```python
from build123d import *

# Parameters (mm, degrees)
SKETCH008_W     = 110
SKETCH008_H     = 66
PAD006_DEPTH    = 2
SKETCH010_W     = 110
SKETCH010_H     = 66
PAD008_DEPTH    = 40
SKETCH011_W     = 106
SKETCH011_H     = 62
POCKET003_DEPTH = 40
SKETCH012_W     = 8
SKETCH012_H     = 8
PAD009_DEPTH    = 38
FILLET_R        = 2
FILLET001_R     = 2
FILLET002_R     = 2
FILLET003_R     = 2
FILLET004_R     = 2
SKETCH009_R     = 3
PAD010_DEPTH    = 10
SKETCH013_W     = 16
SKETCH013_H     = 10
POCKET004_DEPTH = 2
SKETCH014_R     = 1
POCKET005_DEPTH = 8
FILLET005_R     = 1
FILLET006_R     = 1
FILLET007_R     = 2
SKETCH015_R     = 1
POCKET006_DEPTH = 5
FILLET008_R     = 1
SKETCH016_W     = 12
SKETCH016_H     = 2
PAD011_DEPTH    = 38


with BuildPart() as part:
    # Sketch008 → Pad006 (new body)
    with BuildSketch(Plane.XY):
        with Locations((9, 0)):
            Rectangle(SKETCH008_W, SKETCH008_H)
    extrude(amount=PAD006_DEPTH)

    # Sketch010 (on Face6 of Pad006) → Pad008 (join)
    with BuildSketch(Plane.XY.offset(2)):
        with Locations((9, 0)):
            Rectangle(SKETCH010_W, SKETCH010_H)
    extrude(amount=PAD008_DEPTH)

    # Sketch011 (on Face9 of Pad008) → Pocket003 (cut)
    with BuildSketch(Plane.XY.offset(42)):
        with Locations((9, 0)):
            Rectangle(SKETCH011_W, SKETCH011_H)
    extrude(amount=-POCKET003_DEPTH, mode=Mode.SUBTRACT)

    # Sketch012 (on Face15 of Pocket003) → Pad009 (join)
    with BuildSketch(Plane.XY.offset(2)):
        with Locations((-40, 27)):
            Rectangle(SKETCH012_W, SKETCH012_H)
        with Locations((58, 27)):
            Rectangle(SKETCH012_W, SKETCH012_H)
        with Locations((-40, -27)):
            Rectangle(SKETCH012_W, SKETCH012_H)
        with Locations((58, -27)):
            Rectangle(SKETCH012_W, SKETCH012_H)
    extrude(amount=PAD009_DEPTH)

    # Fillet
    fillet_edges = [part.edges().sort_by_distance(p)[0] for p in [
        (62, -31, 41),
    ]]
    fillet(fillet_edges, radius=FILLET_R)

    # Fillet001
    fillet001_edges = [part.edges().sort_by_distance(p)[0] for p in [
        (-44, 31, 41),
    ]]
    fillet(fillet001_edges, radius=FILLET001_R)

    # Fillet002
    fillet002_edges = [part.edges().sort_by_distance(p)[0] for p in [
        (62, 31, 41),
    ]]
    fillet(fillet002_edges, radius=FILLET002_R)

    # Fillet003
    fillet003_edges = [part.edges().sort_by_distance(p)[0] for p in [
        (-44, -31, 41),
    ]]
    fillet(fillet003_edges, radius=FILLET003_R)

    # Fillet004
    fillet004_edges = [part.edges().sort_by_distance(p)[0] for p in [
        (64, 33, 22),
        (64, -33, 22),
        (-46, -33, 22),
        (-46, 33, 22),
    ]]
    fillet(fillet004_edges, radius=FILLET004_R)

    # Sketch009 → Pad010 (join)
    with BuildSketch(Plane.XY.offset(2)):
        with Locations((-38, 18.5)):
            Circle(SKETCH009_R)
        with Locations((45, 18.5)):
            Circle(SKETCH009_R)
        with Locations((-38, -18.5)):
            Circle(SKETCH009_R)
        with Locations((45, -18.5)):
            Circle(SKETCH009_R)
    extrude(amount=PAD010_DEPTH)

    # Sketch013 (on Face5 of Pad010) → Pocket004 (cut)
    with BuildSketch(Plane(origin=(-46, 0, 0), x_dir=(0, -1, 0), z_dir=(-1, 0, 0))):
        with Locations((0, 12)):
            Rectangle(SKETCH013_W, SKETCH013_H)
    extrude(amount=-POCKET004_DEPTH, mode=Mode.SUBTRACT)

    # Sketch014 (on Face35 of Pocket004) → Pocket005 (cut)
    with BuildSketch(Plane.XY.offset(40)):
        with Locations((-40, 27)):
            Circle(SKETCH014_R)
        with Locations((58, 27)):
            Circle(SKETCH014_R)
        with Locations((-40, -27)):
            Circle(SKETCH014_R)
        with Locations((58, -27)):
            Circle(SKETCH014_R)
    extrude(amount=-POCKET005_DEPTH, mode=Mode.SUBTRACT)

    # Fillet005
    fillet005_edges = [part.edges().sort_by_distance(p)[0] for p in [
        (9, 33, 42),
        (63.414214, 32.414214, 42),
        (64, 0, 42),
        (-45.414214, 32.414214, 42),
        (-46, 0, 42),
        (-45.414214, -32.414214, 42),
        (9, -33, 42),
        (63.414214, -32.414214, 42),
    ]]
    fillet(fillet005_edges, radius=FILLET005_R)

    # Fillet006
    fillet006_edges = [part.edges().sort_by_distance(p)[0] for p in [
        (-45, -8, 17),
        (-45, 8, 7),
        (-45, 8, 17),
        (-45, -8, 7),
    ]]
    fillet(fillet006_edges, radius=FILLET006_R)

    # Fillet007
    fillet007_edges = [part.edges().sort_by_distance(p)[0] for p in [
        (54, 23, 21),
        (54, -23, 21),
        (-36, 23, 21),
        (-36, -23, 21),
    ]]
    fillet(fillet007_edges, radius=FILLET007_R)

    # Sketch015 (on Face55 of Fillet007) → Pocket006 (cut)
    with BuildSketch(Plane.XY.offset(12)):
        with Locations((-38, 18.5)):
            Circle(SKETCH015_R)
        with Locations((45, 18.5)):
            Circle(SKETCH015_R)
        with Locations((-38, -18.5)):
            Circle(SKETCH015_R)
        with Locations((45, -18.5)):
            Circle(SKETCH015_R)
    extrude(amount=-POCKET006_DEPTH, mode=Mode.SUBTRACT)

    # Fillet008
    fillet008_edges = [part.edges().sort_by_distance(p)[0] for p in [
        (-46, 8, 12),
        (-46, 7.707107, 7.292893),
        (-46, 7.707107, 16.707107),
        (-46, 0, 17),
        (-46, -7.707107, 16.707107),
        (-46, -8, 12),
        (-46, -7.707107, 7.292893),
        (-46, 0, 7),
    ]]
    fillet(fillet008_edges, radius=FILLET008_R)

    # Sketch016 (on Face21 of Fillet008) → Pad011 (join)
    with BuildSketch(Plane.XY.offset(2)):
        with Locations((9, 30)):
            Rectangle(SKETCH016_W, SKETCH016_H)
        with Locations((9, -30)):
            Rectangle(SKETCH016_W, SKETCH016_H)
    extrude(amount=PAD011_DEPTH)


solid = part.part
```
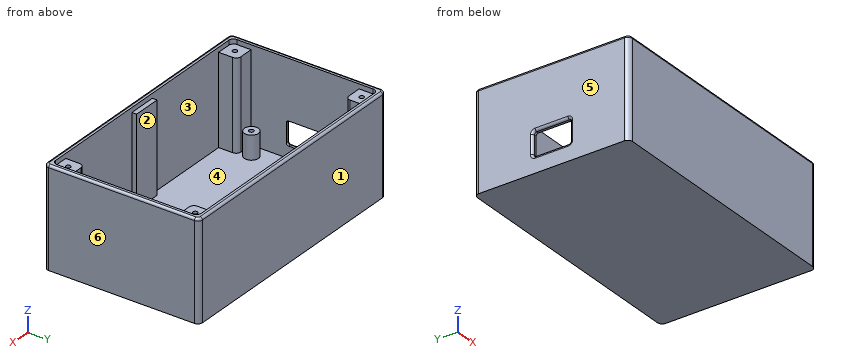
Work out the finished part from the listing and answer in its coordinate system (mm). Face numbers are marked on the shaded views. A direction names the side the tool comes from. Round coordinates to 2 decimals unless told otherwise and drop trailing zeros. Loops run counter-clockwise (first coordinate to the right, second up) from the corner with the lowest first, then second, coordinate; pieces in that order, holes last. Notation, with made-up numbers: (-23, 13) -> (21, 13) arc R31 ccw to (21, 46) -> close; hole circle Ø2 at (66.25, 49.25). An arc over 180 degrees is marked (long way). Write each question's results on one line, items separated by ' | '. Start each with the question number.
1. A tool of negligible diameter and unlimited length cuts with its end or side. For the marked faces 1 and 2, from which of +Z, -Z, +X, -X, +Y, -Y can it reach the whole face along a straight path? Write none if from no direction.
2. Section B-B (x = 32.5) is taken. Determine the outline of the cut face in (y, z), plus the area to 3 significant figures.
3. Find the intervals of material crossed by probe 1 along Y at (x, z) = (45, 8.2); probe 2 along Y at (x, z) = (58, 35); probe 3 along X at (y, z) = (-0.5, 29), in increasing order. Write a range as from..to.
4. Section C-C (z = 4) is taken. State how many separate pieces and enclosed holes the cut face has, plus the area to 3 significant figures.
5. For a pull along X with two mould halves and no side action, classify the marked faces 3, 4, 5 and 6 as +X half, -X half, draft (parallel to the pull), parting line (faces both ways), or undercut.
6. Section D-D (x = 12) is taken. Determine the outline of the cut face in (y, z).
7. Given pin 1 Ø1 at (x, y) = (11.5, -30) entering from +Z; pin 2 Ø1.6 at (x, y) = (-38, 18.5) entering from +Z; pin 3 Ø12 at (x, y) = (-29, -23) entering from -Z; pin 4 Ø2 at (x, y) = (16, -25.5) entering from +Z, each flat-ended and moving along its own axis, determine where each tip first touches the part or whether it passes through.
Evaluation:
1) face 1: +Z, -Z, +X, -X, +Y | face 2: +Z
2) outline: (-33, 0) -> (33, 0) -> (33, 41) arc R1 ccw to (32, 42) -> (31, 42) -> (31, 2) -> (-31, 2) -> (-31, 42) -> (-32, 42) arc R1 ccw to (-33, 41) -> close | area: 292 mm2
3) probe 1: y = -33..-31, -21.5..-19.5, -17.5..-15.5, 15.5..17.5, 19.5..21.5, 31..33 | probe 2: y = -33..-28, -26..-23, 23..26, 28..33 | probe 3: x = -46..-44, 62..64
4) separate pieces: 5 | enclosed holes: 1 | area: 1,100 mm2
5) face 3: undercut | face 4: undercut | face 5: -X half | face 6: +X half
6) outline: (-33, 0) -> (33, 0) -> (33, 41) arc R1 ccw to (32, 42) -> (31, 42) -> (31, 40) -> (29, 40) -> (29, 2) -> (-29, 2) -> (-29, 40) -> (-31, 40) -> (-31, 42) -> (-32, 42) arc R1 ccw to (-33, 41) -> close
7) pin 1: stops at z = 40 | pin 2: stops at z = 7 | pin 3: stops at z = 0 | pin 4: stops at z = 2
